from build123d import *

# Parameters (mm, degrees)
SKETCH_1_R          = 19.1
EXTRUDE_1_DEPTH     = 25.7
SKETCH_1_7_R        = 2
CUT_EXTRUDE_1_DEPTH = 2
CUT_EXTRUDE_2_DEPTH = 38.28417895
CUT_EXTRUDE_3_DEPTH = 21.7
EXTRUDE_START       = 4
SKETCH_1_8_R        = 7.5
EXTRUDE_2_DEPTH     = 21.7
EXTRUDE_3_DEPTH     = 21.7


with BuildPart() as part:
    # 草图1 → 凸台-拉伸1 (new body)
    with BuildSketch(Plane(origin=(0, 0, 0), x_dir=(1, 0, 0), z_dir=(0, 1, 0))):
        with Locations(Location((0, 0, 0), (0, 0, 90))):
            Circle(SKETCH_1_R)
    extrude(amount=EXTRUDE_1_DEPTH)

    # 草图1<7> → 切除-拉伸1 (cut)
    with BuildSketch(Plane(origin=(0, 0, 0), x_dir=(1, 0, 0), z_dir=(0, 1, 0))):
        with Locations((3.535533906, 3.535533906)):
            Circle(SKETCH_1_7_R)
        Polygon((13.435028843, 14.849242405), (2.828427125, 4.242640687), (4.242640687, 2.828427125), (14.849242405, 13.435028843), align=None)
    extrude(amount=CUT_EXTRUDE_1_DEPTH, mode=Mode.SUBTRACT)

    # 草图2 → 切除-拉伸2 (cut, through all)
    with BuildSketch(Plane.XZ):
        with BuildLine():
            Line((12.091525958, 12.091525958), (18.108169541, 6.074882376))
            ThreePointArc((18.108169541, 6.074882376), (13.505739521, 13.505739521), (6.074882376, 18.108169541))
            Line((6.074882376, 18.108169541), (12.091525958, 12.091525958))
        make_face()
        with BuildLine():
            ThreePointArc((-18.108169541, -6.074882376), (-13.505739521, -13.505739521), (-6.074882376, -18.108169541))
            Line((-6.074882376, -18.108169541), (-12.091525958, -12.091525958))
            Line((-12.091525958, -12.091525958), (-18.108169541, -6.074882376))
        make_face()
    extrude(amount=-CUT_EXTRUDE_2_DEPTH, mode=Mode.SUBTRACT)

    # 草图3 → 切除-拉伸3 (cut)
    with BuildSketch(Plane(origin=(0, 25.7, 0), x_dir=(1, 0, 0), z_dir=(0, 1, 0))):
        with BuildLine():
            ThreePointArc((17.1, 0), (10.170102826, 13.74696361), (-5.002808012, 16.35181678))
            Line((-5.002808012, 16.35181678), (-16.35181678, 5.002808012))
            ThreePointArc((-16.35181678, 5.002808012), (-12.091525958, -12.091525958), (5.002808012, -16.35181678))
            Line((5.002808012, -16.35181678), (16.35181678, -5.002808012))
            ThreePointArc((16.35181678, -5.002808012), (16.911919863, -2.529222516), (17.1, 0))
        make_face()
    extrude(amount=-CUT_EXTRUDE_3_DEPTH, mode=Mode.SUBTRACT)

    # 草图1<8> → 凸台-拉伸2 (add)
    with BuildSketch(Plane(origin=(0, 0, 0), x_dir=(1, 0, 0), z_dir=(0, 1, 0)).offset(EXTRUDE_START)):
        with Locations(Location((0, 0, 0), (0, 0, 270))):
            Circle(SKETCH_1_8_R)
        with BuildLine():
            Line((-3.324154028, 2.4), (3.324154028, 2.4))
            ThreePointArc((3.324154028, 2.4), (0, -4.1), (-3.324154028, 2.4))
        make_face(mode=Mode.SUBTRACT)
    extrude(amount=EXTRUDE_2_DEPTH)

    # 草图4 → 拉伸-薄壁3 (add)
    with BuildSketch(Plane(origin=(0, 25.7, 0), x_dir=(1, 0, 0), z_dir=(0, 1, 0))):
        Polygon((-11.384419177, 9.970205615), (-4.313351365, 2.899137803), (-2.899137803, 4.313351365), (-9.970205615, 11.384419177), align=None)
        Polygon((11.384419177, 12.798632739), (3.606244584, 5.020458146), (5.020458146, 3.606244584), (12.798632739, 11.384419177), align=None)
        Polygon((-5.020458146, -3.606244584), (-12.798632739, -11.384419177), (-11.384419177, -12.798632739), (-3.606244584, -5.020458146), align=None)
        Polygon((2.899137803, -4.313351365), (9.970205615, -11.384419177), (11.384419177, -9.970205615), (4.313351365, -2.899137803), align=None)
    extrude(amount=-EXTRUDE_3_DEPTH)


solid = part.part
The listing builds one solid part. Answer for the finished solid, in the listing's coordinates (mm). A direction names the side the tool comes from. Round coordinates to 2 decimals unless told otherwise and drop trailing zeros. Write each loop counter-clockwise with the first axis right and the second up, starting at its lowest first coordinate (ties: lowest second). Pieces come first, ordered by that corner, then holes. Notation, with made-up numbers: M 33.25,25 L 47.25,25 A22 cw 47.25,47 Z; hole C 35,-37 d9. An arc over 180 degrees is marked long. Write each question's results on one line, items separated by ' | '. Start each with the question number.
(1) Determine the mould class of faces 1 (the flat face through (0, 25.7, -3)), 2 (the flat face through (-8.004, 15.002, 9.418)), 3 (the cylindrical face through (-0.1, 14.7, 7.5)) for opening direction X: +X half, -X half, draft (parallel to the pull), parting line (faces both ways), or undercut.
(2) The part is cut by section D-D, the plane z = 10.5. Write down the section's boundary in (x, y), and give its area (3 significant figures).
(3) Find the intervals of material crossed by line 1 (X direction, y = 22.5, z = 9.5); line 2 (X direction, y = 22, z = 5), in increasing order.
(4) The part is cut by section B-B, the plane x = 0. Write down the section's boundary in (y, z), and give its area (3 significant figures).
(5) The part is cut by section C-C, the plane z = -10.5. Write down the section's boundary in (x, y), and give its area (3 significant figures).
(6) Each of these flat-tipped pins is pushed along its axis until it touches: P1, Ø1, axis at x = 1.5, z = -12.5, coming from the -Y side; P2, Ø8, axis at y = 3, z = 13, coming from the -X side; P3, Ø1.5, axis at y = 13.5, z = -14.5, coming from the -X side; P4, Ø12, axis at y = 20, z = -8.5, coming from the +X side. Where does it stop, or does it pass through?
(7) The part is cut by section A-A, the plane y = 19.25. Write down the section's boundary in (x, z), and give its area (3 significant figures).
(8) For faces 4 (the flat face through (7, 2, -7)), 5 (the cylindrical face through (0.1, 14.7, 4.1)), determine the directions among +Z, -Z, +X, -X, +Y, -Y from which every point of the face is accessible in a straight line to the end or side of a thin tool.
Worked answers:
1) face 1: draft | face 2: undercut | face 3: undercut
2) outline: M -15.95,0 L 13.68,0 L 13.68,25.7 L 9.09,25.7 L 9.09,4 L -9.09,4 L -9.09,25.7 L -11.91,25.7 L -11.91,4 L -13.5,4 L -13.5,25.7 L -15.95,25.7 Z | area: 333 mm²
3) line 1: x = -16.57 to -14.22, -10.91 to -8.09, 8.09 to 10.91, 11.85 to 14.68 | line 2: x = -18.43 to -16.35, -6.41 to 6.41, 16.35 to 18.43
4) outline: M 0,-19.1 L 25.7,-19.1 L 25.7,-17.1 L 4,-17.1 L 4,-7.5 L 25.7,-7.5 L 25.7,-2.4 L 4,-2.4 L 4,4.1 L 25.7,4.1 L 25.7,7.5 L 4,7.5 L 4,17.1 L 25.7,17.1 L 25.7,19.1 L 0,19.1 Z | area: 424 mm²
5) outline: M -13.68,0 L 9.09,0 L 9.09,2 L 11.91,2 L 11.91,0 L 15.95,0 L 15.95,25.7 L 13.5,25.7 L 13.5,4 L 11.91,4 L 11.91,25.7 L 9.09,25.7 L 9.09,4 L -9.09,4 L -9.09,25.7 L -13.68,25.7 Z | area: 327 mm²
6) P1: stops at y = 0 | P2: stops at x = -16.85 | P3: stops at x = -10.43 | P4: stops at x = 18.94
7) outline: M -18.11,-6.07 L -6.07,-18.11 A19.1 ccw 18.11,6.07 L 6.07,18.11 A19.1 ccw Z; hole M -16.35,-5 L -11.38,-9.97 L -5.96,-4.55 A7.5 cw -5.96,4.55 L -12.78,11.36 A17.1 ccw Z; hole M -11.36,12.78 L -4.55,5.96 A7.5 cw 4.55,5.96 L 9.97,11.38 L 5,16.35 A17.1 ccw Z; hole M -9.97,-11.38 L -5,-16.35 A17.1 ccw 11.36,-12.78 L 4.55,-5.96 A7.5 cw -4.55,-5.96 Z; hole M -3.32,-2.4 L 3.32,-2.4 A4.1 ccw long Z; hole M 5.96,-4.55 L 12.78,-11.36 A17.1 ccw 16.35,5 L 11.38,9.97 L 5.96,4.55 A7.5 cw Z | area: 426 mm²
8) face 4: -Y | face 5: +Y
